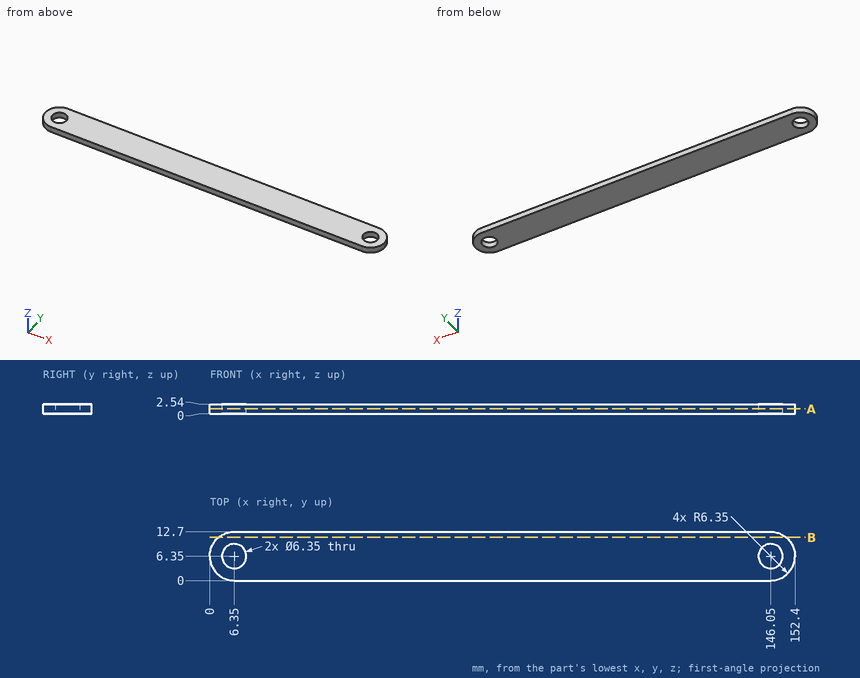
Answer from the drawing. Dimensions are ordinates in mm from the lowest x, y and z of the part. Coordinates: 2 decimals unless noted, no trailing zeros. Write each loop counter-clockwise with the first axis right and the second up, starting at its lowest first coordinate (ties: lowest second). Pieces come first, ordered by that corner, then holes. Notation, with made-up numbers: M 24.25,16.5 L 48.25,16.5 A19 cw 48.25,28.5 Z; hole C 77.5,63.25 d7. An arc over 180 degrees is marked long. Write item = value, one per line.
1. The part is cut by section A-A (z = 1.25). State how many separate pieces and enclosed holes the cut face has, then the cut area to 3 significant figures.
Solution:
separate_pieces = 1
enclosed_holes = 2
area = 1,840 mm2
2. The part is cut by section B-B (y = 11.25). Determine the outline of the cut face in (x, z).
Solution:
outline = M 2.31,0 L 150.09,0 L 150.09,2.54 L 2.31,2.54 Z
3. Flat-ended cylindrical pins translate along their axes: pin 1 (5 mm diameter, centred on x = 6.35, y = 6.35, fed in from -Z); pin 2 (1.5 mm diameter, centred on y = 3, z = 1.5, fed in from -X). Find the tip coordinate at first contact, or state that the pin passes through.
Solution:
pin_1 = through
pin_2 = 0.56
4. Straight lines are drawn through the part: line 1 (X direction, y = 6.75, z = 2.35); line 2 (Y direction, x = 6.35, z = 0.7) (3 decimals); line 3 (X direction, y = 8.25, z = 1.15). For each, find the intervals that lie inside material, in ascending order. Write a range as from..to.
Solution:
line_1 = 0.01..3.2, 9.5..142.9, 149.2..152.39
line_2 = 0..3.175, 9.525..12.7
line_3 = 0.29..3.81, 8.89..143.51, 148.59..152.11
